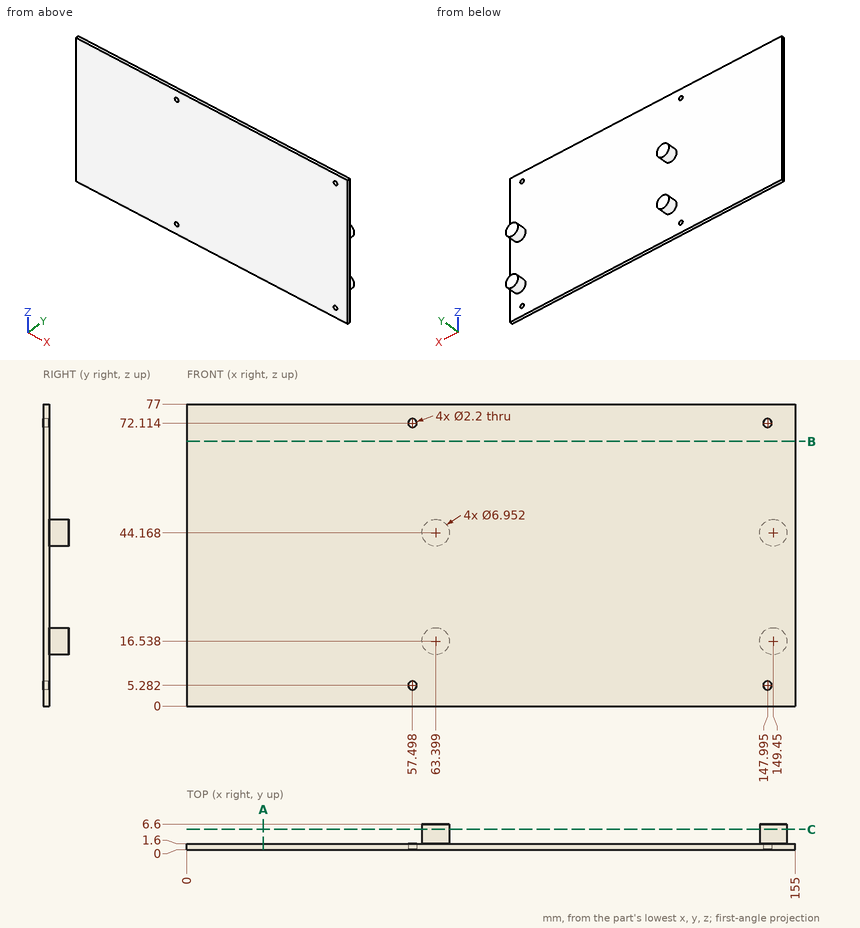
Print and shaded views of the part. All mm, measured from the part's lowest x, y and z. Give positions to 0.01 mm unless a question says otherwise; leave off trailing zeros. Write each loop counter-clockwise with the first axis right and the second up, starting at its lowest first coordinate (ties: lowest second). Pieces come first, ordered by that corner, then holes. Notation, with made-up numbers: (22, 7.25) -> (56, 7.25) arc R25 cw to (56, 34.25) -> close; hole circle Ø1 at (86.25, 2.25). An arc over 180 degrees is marked (long way). Use CSV: the item, a comma, the result in double quotes. Start each with the question number.
1) Drill centre lines: L1, parallel to X at y = 4.75, z = 44; L2, parallel to Y at x = 67, z = 29.5; L3, parallel to Z at x = 62.5, y = 3 (1 decimal). Where is each one in solid material? Low to high.
2) Cut at B-B on z = 67.5. List the corners of the cut face in (x, y), plus the area to 3 significant figures.
3) Cut at C-C on y = 5.25. Count the separate pieces of the cut face and the enclosed holes in it, plus the area to 3 significant figures.
4) Pin check, flat tips, straight feed: P1, Ø2, axis at x = 38.5, y = 4.5, coming from the -Z side; P2, Ø3.5, axis at x = 57.5, z = 5.28, coming from the +Y side. Stop position of each tip, or through.
5) Cut at A-A on x = 19.5. List the corners of the cut face in (y, z).
Final values:
1,L1,"x = 59.93 to 66.87, 145.98 to 152.92"
1,L2,"y = 0 to 1.6"
1,L3,"z = 13.2 to 19.9, 40.8 to 47.5"
2,outline,"(0, 0) -> (155, 0) -> (155, 1.6) -> (0, 1.6) -> close"
2,area,"248 mm2"
3,separate pieces,"4"
3,enclosed holes,"0"
3,area,"152 mm2"
4,P1,"passes through"
4,P2,"stops at y = 1.6"
5,outline,"(0, 0) -> (1.6, 0) -> (1.6, 77) -> (0, 77) -> close"
